Study the drawing (mm; zero at the part's minimum x, y, z) and answer. Coordinates: 2 decimals unless noted, no trailing zeros. Loops run counter-clockwise (first coordinate to the right, second up) from the corner with the lowest first, then second, coordinate; pieces in that order, holes last. Notation, with made-up numbers: (62, 78.5) -> (88, 78.5) arc R23 cw to (88, 90.5) -> close; hole circle Ø3 at (-17.5, 84.5). An arc over 180 degrees is marked (long way). One line per question, with ' | ' between items.
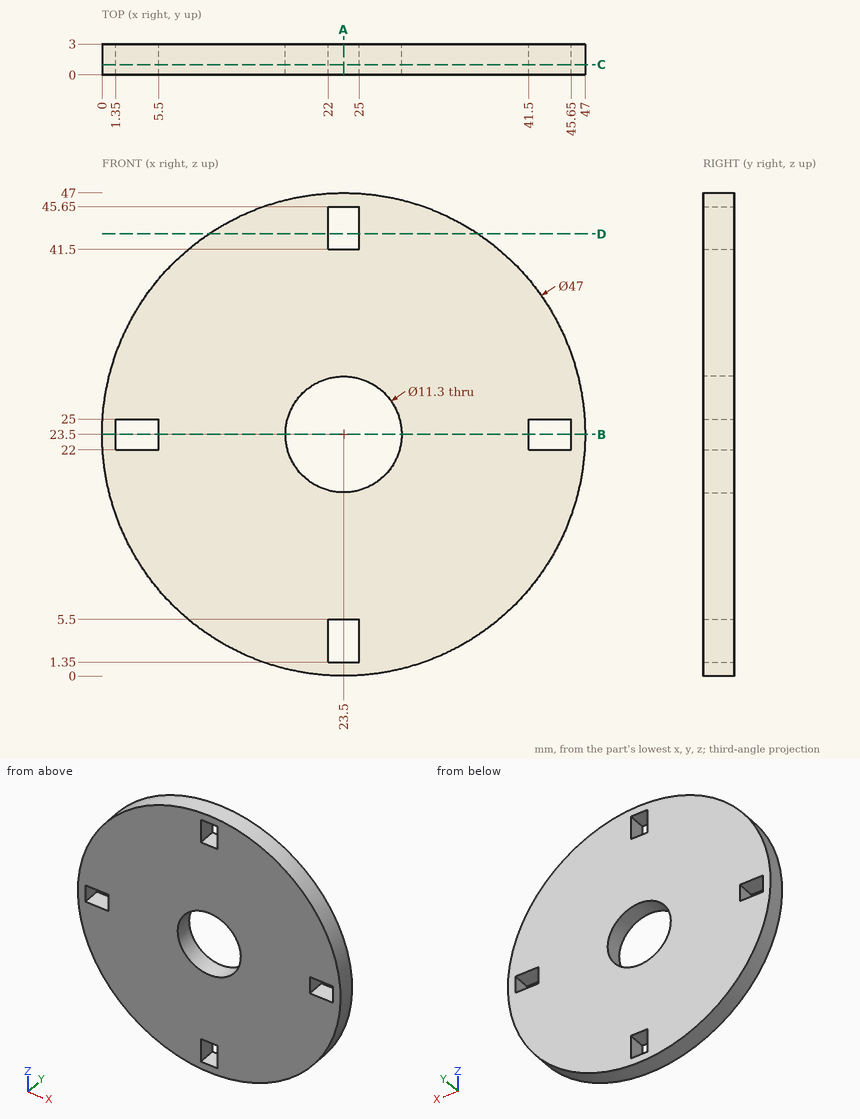
1) Find the intervals of material crossed by line 1 along X through (y, z) = (2.1, 23.5); line 2 along X through (y, z) = (0.9, 44.5); line 3 along Z through (x, y) = (27.5, 0.8), in increasing order.
Check values:
line 1: x = 0 to 1.35, 5.5 to 17.85, 29.15 to 41.5, 45.65 to 47 | line 2: x = 12.95 to 22, 25 to 34.05 | line 3: z = 0.34 to 19.51, 27.49 to 46.66
2) Find section C-C (y = 1). Write down the section's boundary in (x, z).
Check values:
outline: circle Ø47 at (23.5, 23.5); hole (1.35, 22) -> (5.5, 22) -> (5.5, 25) -> (1.35, 25) -> close; hole circle Ø11.3 at (23.5, 23.5); hole (22, 1.35) -> (25, 1.35) -> (25, 5.5) -> (22, 5.5) -> close; hole (22, 41.5) -> (25, 41.5) -> (25, 45.65) -> (22, 45.65) -> close; hole (41.5, 22) -> (45.65, 22) -> (45.65, 25) -> (41.5, 25) -> close
3) Flat-ended cylindrical pins translate along their axes: pin 1 (1 mm diameter, centred on x = 17, y = 1, fed in from +Z); pin 2 (1.5 mm diameter, centred on x = 44, y = 1.5, fed in from -Z); pin 3 (1 mm diameter, centred on y = 0.5, z = 17.5, fed in from +X); pin 4 (10 mm diameter, centred on x = 23.5, z = 23.5, fed in from +Y). Find the tip coordinate at first contact, or state that the pin passes through.
Check values:
pin 1: stops at z = 46.22 | pin 2: stops at z = 10.76 | pin 3: stops at x = 46.35 | pin 4: passes through
4) Find section D-D (z = 43). Write down the section's boundary in (x, y), plus the area to 3 significant figures.
Check values:
outline: (10.39, 0) -> (22, 0) -> (22, 3) -> (10.39, 3) -> close; (25, 0) -> (36.61, 0) -> (36.61, 3) -> (25, 3) -> close | area: 69.7 mm^2
5) Find section B-B (z = 23.5). Write down the section's boundary in (x, y), plus the area to 3 significant figures.
Check values:
outline: (0, 0) -> (1.35, 0) -> (1.35, 3) -> (0, 3) -> close; (5.5, 0) -> (17.85, 0) -> (17.85, 3) -> (5.5, 3) -> close; (29.15, 0) -> (41.5, 0) -> (41.5, 3) -> (29.15, 3) -> close; (45.65, 0) -> (47, 0) -> (47, 3) -> (45.65, 3) -> close | area: 82.2 mm^2
6) Find section A-A (x = 23.5). Write down the section's boundary in (y, z), plus the area to 3 significant figures.
Check values:
outline: (0, 0) -> (3, 0) -> (3, 1.35) -> (0, 1.35) -> close; (0, 5.5) -> (3, 5.5) -> (3, 17.85) -> (0, 17.85) -> close; (0, 29.15) -> (3, 29.15) -> (3, 41.5) -> (0, 41.5) -> close; (0, 45.65) -> (3, 45.65) -> (3, 47) -> (0, 47) -> close | area: 82.2 mm^2
